from build123d import *

# Parameters (mm, degrees)
BOSS_EXTRUDE1_DEPTH = 40


with BuildPart() as part:
    # Sketch1 → Boss-Extrude1 (new body)
    with BuildSketch(Plane.XY):
        with BuildLine():
            Line((0, 15), (0, 0))
            Line((0, 0), (114.35, 0))
            ThreePointArc((114.35, 0), (119.35, 5), (114.35, 10))
            Line((114.35, 10), (78.619624256, 10))
            ThreePointArc((78.619624256, 10), (45.494135139, 20.4444266), (24.35, 48))
            Line((24.35, 48), (14.35, 48))
            Line((14.35, 48), (14.35, 3))
            Line((14.35, 3), (8, 3))
            Line((8, 3), (8, 15))
            ThreePointArc((8, 15), (4, 19), (0, 15))
        make_face()
    extrude(amount=BOSS_EXTRUDE1_DEPTH)


solid = part.part
Can you work these out from the model? Positions are in its coordinate system, mm. A direction names the side the tool comes from. Coordinates: 2 decimals unless noted, no trailing zeros. Loops run counter-clockwise (first coordinate to the right, second up) from the corner with the lowest first, then second, coordinate; pieces in that order, holes last. Notation, with made-up numbers: (46, -10) - (61, -10) arc R18 ccw to (61, -3) - close; hole circle Ø10 at (83.5, 5). An arc over 180 degrees is marked (long way). Answer as a JSON object with one key per item and string values. Group by question number.
Item 1: If we section it at A-A (y = 5): List the corners of the cut face in (x, z) for me.
Item 2: If we section it at B-B (z = 22.5): List the corners of the cut face in (x, y) for me.
Item 3: For pin 1 (12 mm diameter, centred on y = 30.5, z = 24, fed in from -X); pin 2 (2 mm diameter, centred on x = 53.5, z = 13, fed in from +Y); pin 3 (3 mm diameter, centred on x = 44.5, z = 28.5, fed in from +Y), each with a flat end and sliding along its axis, tell me the tip position at first contact or that it passes through.
Item 4: If we section it at D-D (y = 30.5): List the corners of the cut face in (x, z) for me.
Item 5: If I drill on L1, parallel to Y at x = 86, z = 35; L2, parallel to Y at x = 13, z = 11; L3, parallel to X at y = 5, z = 29.5, over which ranges is the centre line in solid material (lowest first)? Write a range as from..to.
Item 6: If we mould it in two halves opening along X, with no side actions, what happens to faces 1 (the face through (45.9, 20.163, 19.72)), 2 (the face through (46, 14, 0)), 3 (the face through (0, 8, 20)), 4 (the face through (11, 3, 20))? For each: released by +X, released by -X, zero draft, split by the parting line, or undercut.
Item 7: On a 3-axis mill with a long thin cutter (end or side, diameter ignored), from which of +Z, -Z, +X, -X, +Y, -Y can I reach the whole of each face in a straight line? I mean faces 5 (the face through (8, 9, 20)), 6 (the face through (46, 14, 40)), 7 (the face through (97, 10, 20)). Say none if no direction works.
Item 8: If we section it at C-C (x = 90.5): List the corners of the cut face in (y, z) for me.
Returned:
{
 "1": {"outline": "(0, 0) - (8, 0) - (8, 40) - (0, 40) - close; (14.35, 0) - (119.35, 0) - (119.35, 40) - (14.35, 40) - close"},
 "2": {"outline": "(0, 0) - (114.35, 0) arc R5 ccw to (114.35, 10) - (78.62, 10) arc R57.75 cw to (24.35, 48) - (14.35, 48) - (14.35, 3) - (8, 3) - (8, 15) arc R4 ccw to (0, 15) - close"},
 "3": {"pin 1": "stops at x = 14.35", "pin 2": "stops at y = 16.24", "pin 3": "stops at y = 22.29"},
 "4": {"outline": "(14.35, 0) - (34.49, 0) - (34.49, 40) - (14.35, 40) - close"},
 "5": {"L1": "y = 0..10", "L2": "y = 0..3", "L3": "x = 0..8, 14.35..119.35"},
 "6": {"face 1": "released by +X", "face 2": "zero draft", "face 3": "released by -X", "face 4": "undercut"},
 "7": {"face 5": "+Z, -Z, +Y", "face 6": "+Z, +X, -X, +Y, -Y", "face 7": "+Z, -Z, +X, +Y"},
 "8": {"outline": "(0, 0) - (10, 0) - (10, 40) - (0, 40) - close"}
}
